Check sheet for the modelled part. Datum: model origin and axes. Units: mm. A direction names the side the tool comes from. Give positions to 0.01 mm unless a question says otherwise; leave off trailing zeros. Write each loop counter-clockwise with the first axis right and the second up, starting at its lowest first coordinate (ties: lowest second). Pieces come first, ordered by that corner, then holes. Notation, with made-up numbers: (49, -11.75) -> (96, -11.75) arc R23 ccw to (96, 2.25) -> close; hole circle Ø4 at (67.25, 38). An arc over 180 degrees is marked (long way). Answer as a JSON object with one key per item and string values.
from build123d import *

# Parameters (mm, degrees)
SKETCH_1_R      = 3.825
SKETCH_1_R_2    = 2.05
SKETCH_1_R_3    = 9.55
SKETCH_1_W      = 8.1
SKETCH_1_H      = 2.1
EXTRUDE_1_DEPTH = 2


with BuildPart() as part:
    # 草图1 → 凸台-拉伸1 (new body)
    with BuildSketch(Plane.XY):
        Polygon((81, -15.149736791), (81, 7.149736791), (40.992999038, 17.149736791), (12.70872779, 17.149736791), (-19, 7.149736791), (-19, -15.149736791), (12.70872779, -25.149736791), (40.992999038, -25.149736791), align=None)
        Circle(SKETCH_1_R, mode=Mode.SUBTRACT)
        with Locations((62, 0)):
            Circle(SKETCH_1_R, mode=Mode.SUBTRACT)
        with Locations((62, -8)):
            Circle(SKETCH_1_R, mode=Mode.SUBTRACT)
        with Locations((0, -8)):
            Circle(SKETCH_1_R, mode=Mode.SUBTRACT)
        with Locations((45.142135624, 10.142135624)):
            Circle(SKETCH_1_R_2, mode=Mode.SUBTRACT)
        with Locations((45.142135624, -18.142135624)):
            Circle(SKETCH_1_R_2, mode=Mode.SUBTRACT)
        with Locations((16.857864376, -18.142135624)):
            Circle(SKETCH_1_R_2, mode=Mode.SUBTRACT)
        with Locations((16.857864376, 10.142135624)):
            Circle(SKETCH_1_R_2, mode=Mode.SUBTRACT)
        with Locations((74, 0)):
            Circle(SKETCH_1_R, mode=Mode.SUBTRACT)
        with Locations((74, -8)):
            Circle(SKETCH_1_R, mode=Mode.SUBTRACT)
        with Locations((-12, -8)):
            Circle(SKETCH_1_R, mode=Mode.SUBTRACT)
        with Locations((-12, 0)):
            Circle(SKETCH_1_R, mode=Mode.SUBTRACT)
        with Locations((31, -4)):
            Circle(SKETCH_1_R_3, mode=Mode.SUBTRACT)
        with Locations((15, 0)):
            Rectangle(SKETCH_1_W, SKETCH_1_H, mode=Mode.SUBTRACT)
        with Locations((47, 0)):
            Rectangle(SKETCH_1_W, SKETCH_1_H, mode=Mode.SUBTRACT)
        with Locations((47, -8)):
            Rectangle(SKETCH_1_W, SKETCH_1_H, mode=Mode.SUBTRACT)
        with Locations((15, -8)):
            Rectangle(SKETCH_1_W, SKETCH_1_H, mode=Mode.SUBTRACT)
    extrude(amount=EXTRUDE_1_DEPTH)


solid = part.part
1. Sectioned sample at D-D, the plane y = 9. Enter the section's corners in (x, z), plus the area to 3 significant figures.
Determined:
{"outline": "(-13.13, 0) -> (15.16, 0) -> (15.16, 2) -> (-13.13, 2) -> close; (18.56, 0) -> (43.44, 0) -> (43.44, 2) -> (18.56, 2) -> close; (46.84, 0) -> (73.6, 0) -> (73.6, 2) -> (46.84, 2) -> close", "area": "160 mm^2"}
2. Mould release check, pull along Y, two halves, no side actions. Record for faces 1 (the face through (-2.92, 12.22, 0.99)), 2 (the face through (30, 6, 2)), 3 (the face through (47, -6.95, 1)): released by +Y, released by -Y, zero draft, split by the parting line, or undercut.
Determined:
{"face 1": "released by +Y", "face 2": "zero draft", "face 3": "undercut"}
3. Go/stop test with flat-tipped pins: P1, Ø6, axis at x = 56.5, y = 2.5, coming from the -Z side; P2, Ø7, axis at x = 0, y = -8, coming from the -Z side. Record where each tip stops, or that it passes through.
Determined:
{"P1": "z = 0", "P2": "through"}
4. Access from +Z, -Z, +X, -X, +Y, -Y to the whole of each face (thin tool, end or side, straight path). Record for faces 4 (the face through (60.72, -20.22, 0.99)), 5 (the face through (47, 1.05, 1)).
Determined:
{"face 4": "+Z, -Z, +X, -Y", "face 5": "+Z, -Z"}
5. Sectioned sample at A-A, the plane x = 31. Enter the section's corners in (y, z).
Determined:
{"outline": "(-25.15, 0) -> (-13.55, 0) -> (-13.55, 2) -> (-25.15, 2) -> close; (5.55, 0) -> (17.15, 0) -> (17.15, 2) -> (5.55, 2) -> close"}
6. Sectioned sample at C-C, the plane x = 62. Enter the section's corners in (y, z) (3 decimals).
Determined:
{"outline": "(-19.899, 0) -> (-11.825, 0) -> (-11.825, 2) -> (-19.899, 2) -> close; (-4.175, 0) -> (-3.825, 0) -> (-3.825, 2) -> (-4.175, 2) -> close; (3.825, 0) -> (11.899, 0) -> (11.899, 2) -> (3.825, 2) -> close"}
7. Scan lines: L1, parallel to Y at x = 17, z = 0.6; L2, parallel to Y at x = 0, z = 0.6 (3 decimals); L3, parallel to Y at x = 1, z = 0.2. Record each from-to range of solid material in increasing order. Write a range as [from, to].
Determined:
{"L1": "[-25.15, -20.19], [-16.1, -9.05], [-6.95, -1.05], [1.05, 8.1], [12.19, 17.15]", "L2": "[-21.142, -11.825], [-4.175, -3.825], [3.825, 13.142]", "L3": "[-21.46, -11.69], [-4.31, -3.69], [3.69, 13.46]"}
8. Sectioned sample at B-B, the plane y = -2. Enter the section's corners in (x, z), plus the area to 3 significant figures.
Determined:
{"outline": "(-19, 0) -> (-15.26, 0) -> (-15.26, 2) -> (-19, 2) -> close; (-8.74, 0) -> (-3.26, 0) -> (-3.26, 2) -> (-8.74, 2) -> close; (3.26, 0) -> (21.66, 0) -> (21.66, 2) -> (3.26, 2) -> close; (40.34, 0) -> (58.74, 0) -> (58.74, 2) -> (40.34, 2) -> close; (65.26, 0) -> (70.74, 0) -> (70.74, 2) -> (65.26, 2) -> close; (77.26, 0) -> (81, 0) -> (81, 2) -> (77.26, 2) -> close", "area": "110 mm^2"}
